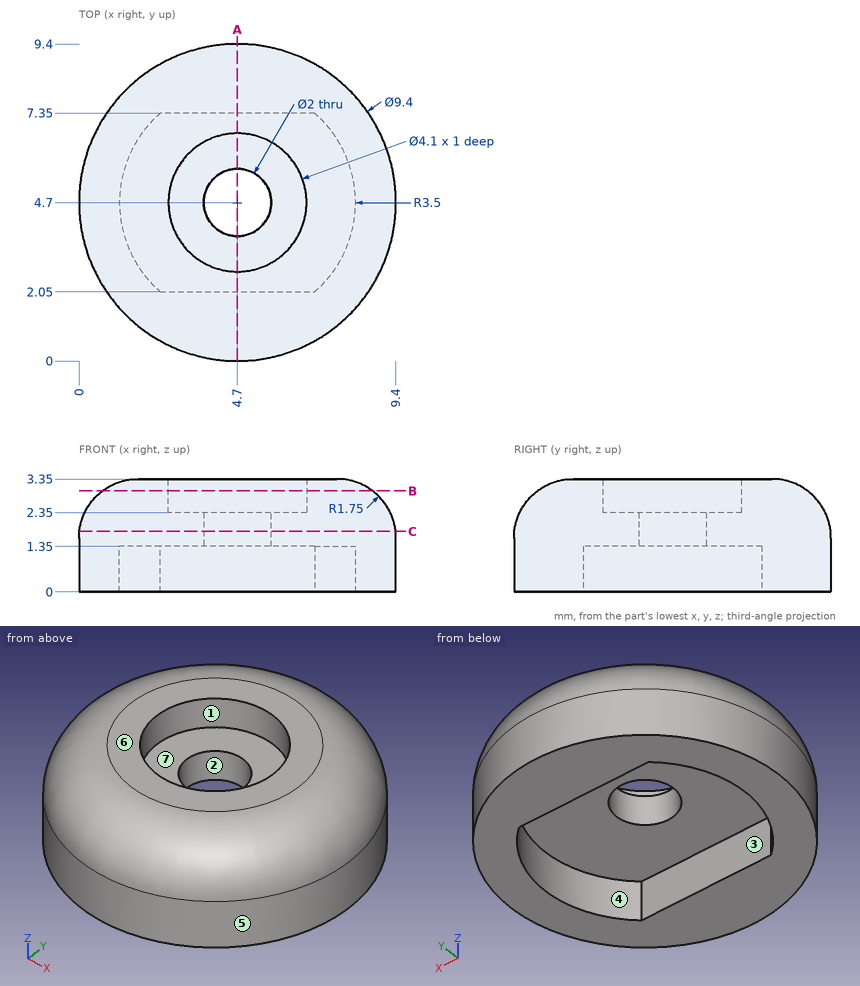
For this review, use the dimensioned drawing (mm, ordinates from the lowest corner) and the shaded views. A direction names the side the tool comes from. Round coordinates to 2 decimals unless told otherwise and drop trailing zeros. Write each loop counter-clockwise with the first axis right and the second up, starting at its lowest first coordinate (ties: lowest second). Pieces come first, ordered by that corner, then holes. Notation, with made-up numbers: (-24, -34.75) - (-7, -34.75) arc R13 ccw to (-7, -19.75) - close; hole circle Ø1 at (-39.75, 62.5). An arc over 180 degrees is marked (long way). Use a Markdown table: item, result.
Q1. We need section A-A (x = 4.7). Give the boundary of the cut face in (y, z), plus the area to 3 significant figures.
Derived:
| item | result |
|---|---|
| outline | (0, 0) - (2.05, 0) - (2.05, 1.35) - (3.7, 1.35) - (3.7, 2.35) - (2.65, 2.35) - (2.65, 3.35) - (1.75, 3.35) arc R1.75 ccw to (0, 1.6) - close; (5.7, 1.35) - (7.35, 1.35) - (7.35, 0) - (9.4, 0) - (9.4, 1.6) arc R1.75 ccw to (7.65, 3.35) - (6.75, 3.35) - (6.75, 2.35) - (5.7, 2.35) - close |
| area | 16.9 mm2 |
Q2. The part is to be moulded in two halves that separate along Y. For the marked faces 4, 5, 6 and 7, say which applies: pulls with the +Y half, pulls with the -Y half, needs draft (parallel to the pull), parting line crosses it, or undercut.
Derived:
| item | result |
|---|---|
| face 4 | undercut |
| face 5 | parting line crosses it |
| face 6 | needs draft |
| face 7 | undercut |
Q3. We need section B-B (z = 3). Give the boundary of the cut face in (x, y).
Derived:
| item | result |
|---|---|
| outline | circle Ø8 at (4.7, 4.7); hole circle Ø4.1 at (4.7, 4.7) |
Q4. Wall thickness on line 1 along Y through (x, z) = (4, 0.65); line 2 along Y through (x, z) = (6.75, 0.9); line 3 along X through (y, z) = (2.5, 0.6): over which ranges is each line inside the solid? List them lowest first.
Derived:
| item | result |
|---|---|
| line 1 | y = 0.05 to 2.05, 7.35 to 9.35 |
| line 2 | y = 0.47 to 2.05, 7.35 to 8.93 |
| line 3 | x = 0.55 to 1.98, 7.42 to 8.85 |
Q5. Machinability: for the marked faces 1, 2 and 3, which of the approach directions +Z, -Z, +X, -X, +Y, -Y give a long, thin tool a straight path to every point of the face, cutting with its end or side? Answer none if there is none.
Derived:
| item | result |
|---|---|
| face 1 | +Z |
| face 2 | +Z, -Z |
| face 3 | -Z |
Q6. We need section C-C (z = 1.8). Give the boundary of the cut face in (x, y).
Derived:
| item | result |
|---|---|
| outline | circle Ø9.38 at (4.7, 4.7); hole circle Ø2 at (4.7, 4.7) |
Q7. Clearance check with flat-ended pins moving along their axes: pin 1 (0.7 mm diameter, centred on x = 3.5, z = 0.5, fed in from +Y); pin 2 (1.5 mm diameter, centred on y = 6.5, z = 3, fed in from +X); pin 3 (1.6 mm diameter, centred on x = 4.7, y = 4.7, fed in from +Z); pin 4 (2 mm diameter, centred on x = 4, y = 5, fed in from +Z). State where each tip first meets the part, or that it passes through.
Derived:
| item | result |
|---|---|
| pin 1 | stops at y = 9.32 |
| pin 2 | stops at x = 9 |
| pin 3 | passes through |
| pin 4 | stops at z = 2.35 |
